Source: three-view drawing plus pictorial views. Frame: mm from the lowest corner of the part. A direction names the side the tool comes from. Give positions to 0.01 mm unless a question says otherwise; leave off trailing zeros. Loops run counter-clockwise (first coordinate to the right, second up) from the corner with the lowest first, then second, coordinate; pieces in that order, holes last. Notation, with made-up numbers: (73.25, 12) -> (100.25, 12) arc R18 ccw to (100.25, 35) -> close; hole circle Ø9 at (-20.75, 7.5). An arc over 180 degrees is marked (long way). One line per item, written item: value. Start each with the question number.
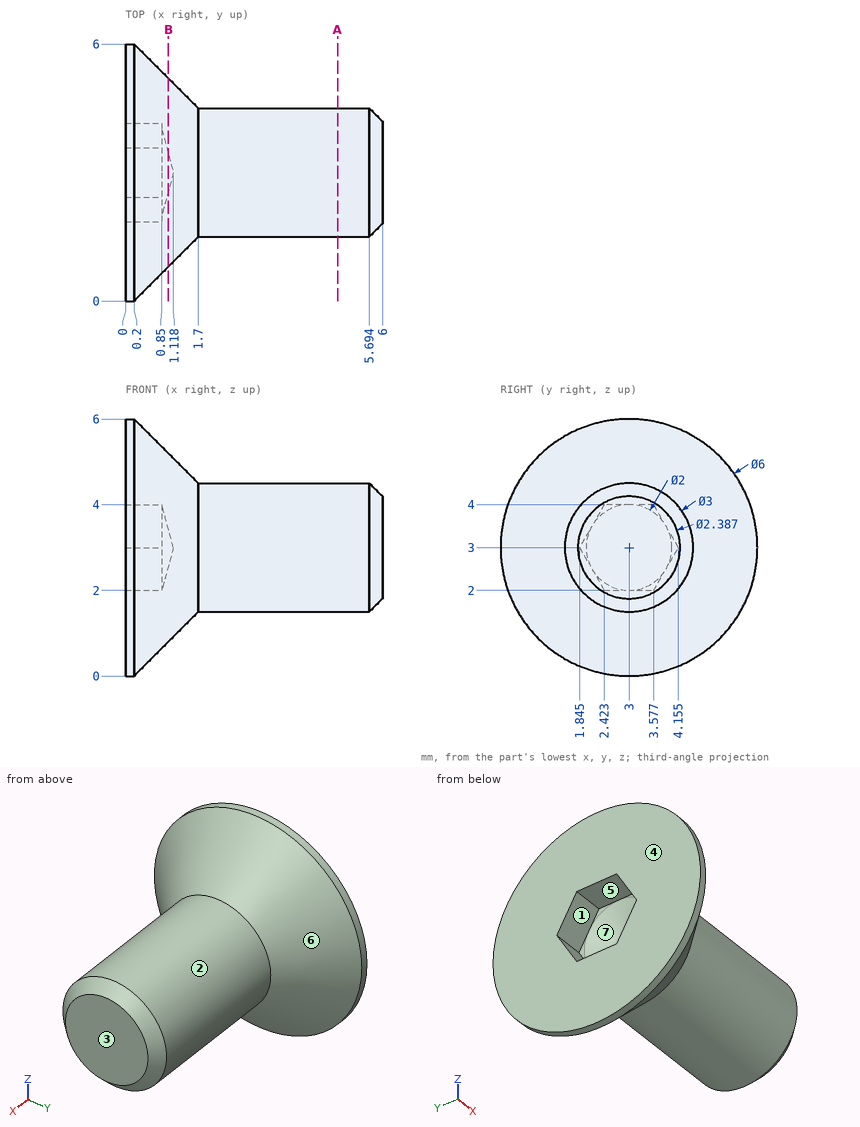
Item 1: Section A-A, the plane x = 4.95. Output: boundary loops of the cut face in (y, z).
Item 2: Pin query (flat end, axial travel): pin 1 (1.3 mm diameter, centred on y = 3.5, z = 3, fed in from -X); pin 2 (1.5 mm diameter, centred on x = 5, z = 1.5, fed in from +Y). Return the tip coordinate at first contact, or that it passes through.
Item 3: Mould query, pull axis Y, two halves, no side actions, for the marked faces 4, 5, 6 and 7. Classes: pulls with the +Y half, pulls with the -Y half, needs draft (parallel to the pull), parting line crosses it, or undercut.
Item 4: Section B-B, the plane x = 1. Output: boundary loops of the cut face in (y, z), then the cut area to 3 significant figures.
Item 5: Ray query, line 1 along Y through (x, z) = (0.5, 2.1) (1 decimal); line 2 along Z through (x, y) = (5.1, 2); line 3 along Z through (x, y) = (4.7, 2.55). Return the intervals inside material, ascending. Write a range as [from, to].
Item 6: Access query for the marked faces 1, 2 and 3. Directions: +Z, -Z, +X, -X, +Y, -Y. A direction counts if a zero-diameter tool reaches every point of the face in a straight line with its end or side. Return the directions, or none.
Geometry check:
1. outline: circle Ø3 at (3, 3)
2. pin 1: stops at x = 0
2. pin 2: stops at y = 4.3
3. face 4: needs draft
3. face 5: undercut
3. face 6: parting line crosses it
3. face 7: undercut
4. outline: circle Ø4.4 at (3, 3); hole circle Ø0.88 at (3, 3)
4. area: 14.6 mm2
5. line 1: y = [0.5, 2.4], [3.6, 5.5]
5. line 2: z = [1.88, 4.12]
5. line 3: z = [1.57, 4.43]
6. face 1: -X
6. face 2: +X
6. face 3: +Z, -Z, +X, +Y, -Y
